Design review of the part built by this model. Coordinates are the model's own, in mm. Face numbers are marked on the shaded views. Coordinates: 2 decimals unless noted, no trailing zeros. Answer as a JSON object with one key per item and string values.
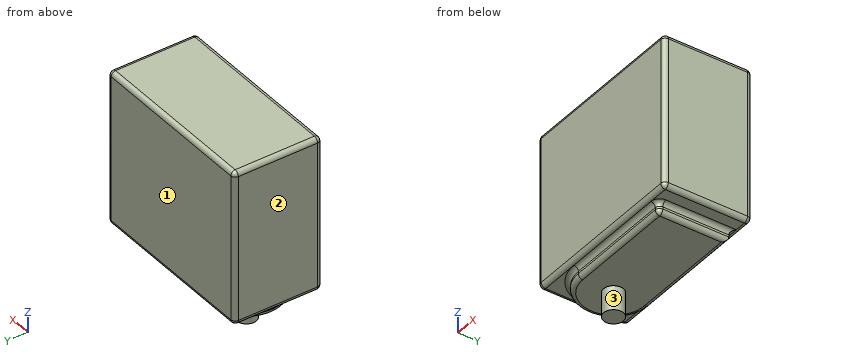
from build123d import *

# Parameters (mm, degrees)
SKETCH_1_W      = 40
SKETCH_1_H      = 20
EXTRUDE_1_DEPTH = 35
FILLET_1_R      = 1
SKETCH_2_R      = 2.240395976
EXTRUDE_2_DEPTH = 8
EXTRUDE_3_DEPTH = 2.5
FILLET_2_R      = 1


with BuildPart() as part:
    # 草图1 → 凸台-拉伸1 (new body)
    with BuildSketch(Plane.XY):
        Rectangle(SKETCH_1_W, SKETCH_1_H)
    extrude(amount=EXTRUDE_1_DEPTH)

    # 圆角1
    fillet_1_edges = [part.edges().sort_by_distance(p)[0] for p in [
        (-20, 0, 35),
        (0, -10, 35),
        (20, 0, 35),
        (0, -10, 0),
        (-20, 0, 0),
        (0, 10, 0),
        (20, 0, 0),
        (0, 10, 35),
        (20, -10, 17.5),
        (-20, -10, 17.5),
        (-20, 10, 17.5),
        (20, 10, 17.5),
    ]]
    fillet(fillet_1_edges, radius=FILLET_1_R)

    # 草图2 → 凸台-拉伸2 (add)
    with BuildSketch(Plane(origin=(0, 0, 0), x_dir=(-1, 0, 0), z_dir=(0, 0, -1))):
        with Locations(Location((10, 0, 0), (0, 0, 180))):
            Circle(SKETCH_2_R)
    extrude(amount=EXTRUDE_2_DEPTH)

    # 草图3 → 凸台-拉伸3 (add)
    with BuildSketch(Plane(origin=(0, 0, 0), x_dir=(-1, 0, 0), z_dir=(0, 0, -1))):
        with BuildLine():
            Line((-15.444071046, 8), (-15.444071046, -8))
            Line((-15.444071046, -8), (10, -8))
            ThreePointArc((10, -8), (18, 0), (10, 8))
            Line((10, 8), (-15.444071046, 8))
        make_face()
    extrude(amount=EXTRUDE_3_DEPTH)

    # 圆角2
    fillet_2_edges = [part.edges().sort_by_distance(p)[0] for p in [
        (-18, 0, 0),
        (2.722035523, 8, 0),
        (15.444071046, 0, 0),
        (2.722035523, -8, 0),
        (15.444071046, -8, -1.25),
        (-18, 0, -2.5),
        (2.722035523, 8, -2.5),
        (15.444071046, 0, -2.5),
        (2.722035523, -8, -2.5),
    ]]
    fillet(fillet_2_edges, radius=FILLET_2_R - 0.0001)  # a hair under: the kernel refuses the full size


solid = part.part
1) Mouldability with a two-part tool opening along Y and no side actions: class the marked faces 1, 2 and 3 as released by +Y, released by -Y, zero draft, split by the parting line, or undercut.
Taken from the geometry:
{"face 1": "released by +Y", "face 2": "zero draft", "face 3": "split by the parting line"}
2) To check wall thickness, follow L1, parallel to Z at x = 2, y = -4.25; L2, parallel to Z at x = 17, y = -0.75; L3, parallel to X at y = -0.5, z = -5.5. State the ranges of each line that lie inside material, in increasing order.
Taken from the geometry:
{"L1": "z = -2.5 to 35", "L2": "z = 0 to 35", "L3": "x = -12.18 to -7.82"}
3) Insertion check: pin 1 Ø3 at (x, z) = (-10, -3.5) entering from +Y; pin 2 Ø1 at (x, y) = (4, 5) entering from -Z; pin 3 Ø12 at (x, y) = (-14.5, -6.5) entering from -Z. Each pin has a flat end and moves straight along its axis. Give the tip position at first contact, or say it passes through.
Taken from the geometry:
{"pin 1": "stops at y = 7.87", "pin 2": "stops at z = -2.5", "pin 3": "stops at z = -8"}
